Geometry check sheet. Reference: the model listing, model coordinates, mm. Face numbers are marked on the shaded views. A direction names the side the tool comes from. Give positions to 0.01 mm unless a question says otherwise; leave off trailing zeros. Loops run counter-clockwise (first coordinate to the right, second up) from the corner with the lowest first, then second, coordinate; pieces in that order, holes last. Notation, with made-up numbers: (88.25, 29) -> (130.25, 29) arc R24 ccw to (130.25, 65) -> close; hole circle Ø1 at (73, 79.5). An arc over 180 degrees is marked (long way). Answer in a Markdown table with one row per item. Add a question column.
Solid Edge part; units mm, degrees
sketch "Sketch1" plane through (0, 0, 0) normal (0, 0, 1) x (1, 0, 0)
  circle A0 centre (0, 0) radius 8
extrude "Protrusion1" add sketch "Sketch1" along normal blind 10
sketch "Sketch2" plane through (0, 0, 0) normal (0, 0, -1) x (1, 0, 0)
  circle A0 centre (0, 0) radius 5
extrude "Protrusion2" add sketch "Sketch2" along normal blind 25
sketch "Sketch3" plane through (0, 0, -25) normal (0, 0, -1) x (1, 0, 0)
  circle A0 centre (0, 0) radius 4.9997
extrude "Cutout1" cut sketch "Sketch3" against normal blind 24.975 flip side to cut
chamfer "Chamfer_1" distance 0.75 angle 45 1 edges at (-4.9997, 0, -25)
sketch "Sketch4" plane through (0, 0, 10) normal (0, 0, 1) x (1, 0, 0)
  line L0 (-2.3094, 4) -> (2.3094, 4)
  line L1 (4.6188, 0) -> (2.3094, 4)
  line L2 (2.3094, -4) -> (4.6188, 0)
  line L3 (-2.3094, -4) -> (2.3094, -4)
  line L4 (-4.6188, 0) -> (-2.3094, -4)
  line L5 (-2.3094, 4) -> (-4.6188, 0)
extrude "Cutout2" cut sketch "Sketch4" against normal blind 5
properties part number "24102802"
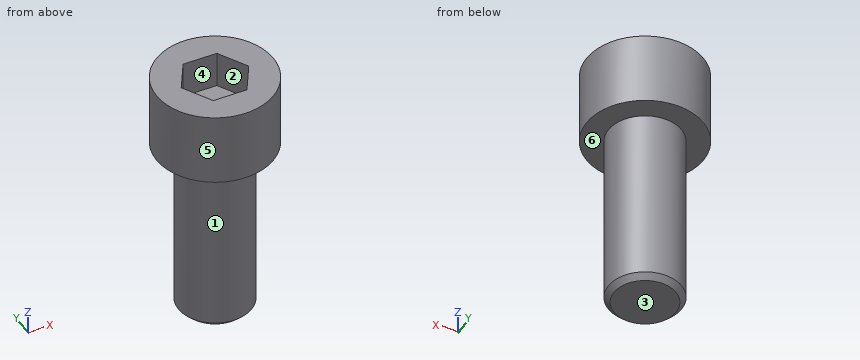
1. Sectioned sample at D-D (y = -6). Enter the section's corners in (x, z).
2. Material ranges on L1, parallel to Z at x = -0.5, y = 3.5; L2, parallel to Z at x = 5.75, y = -1.75; L3, parallel to X at y = 0, z = -9, recorded low to high. Write a range as from..to.
3. Sectioned sample at C-C (z = -0.5). Enter the section's corners in (x, y).
4. Access from +Z, -Z, +X, -X, +Y, -Y to the whole of each face (thin tool, end or side, straight path). Record for the marked faces 4, 5 and 6.
5. Release check for a two-part mould opening along Y. For the marked faces 1, 2 and 3 record: released by +Y, released by -Y, zero draft, split by the parting line, or undercut.
6. Sectioned sample at A-A (z = 7). Enter the section's corners in (x, y).
7. Gauge pin test, flat ends, axial feed: pin 1 Ø3 at (x, z) = (-5, -15) entering from +Y; pin 2 Ø2 at (x, z) = (-1, -14) entering from -Y; pin 3 Ø2 at (x, z) = (-2.5, -8) entering from -Y. Record the tip position at first contact, or that the pin passes through.
Response:
| question | item | result |
|---|---|---|
| 1 | outline | (-5.29, 0) -> (5.29, 0) -> (5.29, 10) -> (-5.29, 10) -> close |
| 2 | L1 | z = -25..5 |
| 2 | L2 | z = 0..10 |
| 2 | L3 | x = -5..5 |
| 3 | outline | circle Ø10 at (0, 0) |
| 4 | face 4 | +Z |
| 4 | face 5 | +Z, -Z |
| 4 | face 6 | -Z |
| 5 | face 1 | split by the parting line |
| 5 | face 2 | undercut |
| 5 | face 3 | zero draft |
| 6 | outline | circle Ø16 at (0, 0); hole (-4.62, 0) -> (-2.31, -4) -> (2.31, -4) -> (4.62, 0) -> (2.31, 4) -> (-2.31, 4) -> close |
| 7 | pin 1 | stops at y = 3.57 |
| 7 | pin 2 | stops at y = -5 |
| 7 | pin 3 | stops at y = -4.77 |
